The model under review builds one solid part; all positions refer to its coordinate system, in mm. Coordinates: 2 decimals unless noted, no trailing zeros. Loops run counter-clockwise (first coordinate to the right, second up) from the corner with the lowest first, then second, coordinate; pieces in that order, holes last. Notation, with made-up numbers: (-13.75, -37) -> (7.25, -37) arc R25 ccw to (7.25, -14) -> close; hole circle Ø3 at (-29, 32.25). An arc over 180 degrees is marked (long way). One line per question, with ' | ' between items. Start each with the question number.
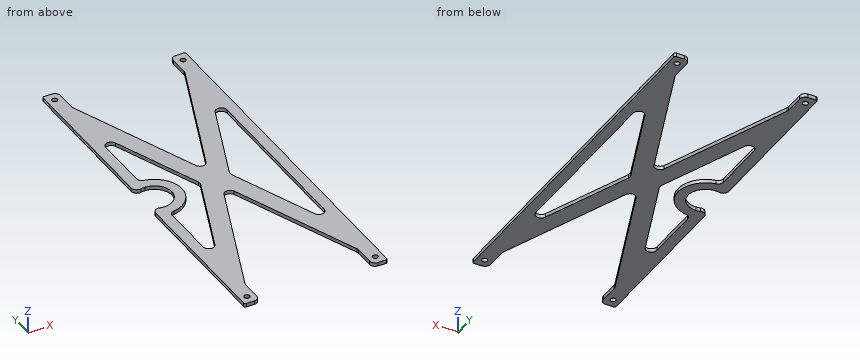
from build123d import *
from build123d.topology import SkipClean

# Parameters (mm, degrees)
EXTRUDE_1_DEPTH     = 2
SKETCH_4_R          = 1.5
CUT_EXTRUDE_3_DEPTH = 108.354552768
FILLET_4_R          = 1
CUT_EXTRUDE_5_DEPTH = 108.354552768
FILLET_7_R          = 3
EXTRUDE_2_DEPTH     = 2
CUT_EXTRUDE_6_DEPTH = 108.354552899
FILLET_8_R          = 3


with BuildPart() as part:
    # 草图1 → 凸台-拉伸1 (new body)
    with BuildSketch(Plane.XY):
        Polygon((39, 79.487179487), (33, 64.102564103), (33, -64.102564103), (39, -79.487179487), align=None)
        Polygon((33, -64.102564103), (8, 0), (0, -20.512820513), (31, -100), (39, -100), (39, -79.487179487), align=None)
        Polygon((-31, -100), (0, -20.512820513), (-8, 0), (-33, -64.102564103), (-39, -79.487179487), (-39, -100), align=None)
        Polygon((-33, -64.102564103), (-33, 64.102564103), (-39, 79.487179487), (-39, -79.487179487), align=None)
        Polygon((0, -20.512820513), (8, 0), (0, 20.512820513), (-8, 0), align=None)
        Polygon((8, 0), (33, 64.102564103), (39, 79.487179487), (39, 100), (31, 100), (0, 20.512820513), align=None)
        Polygon((-8, 0), (0, 20.512820513), (-31, 100), (-39, 100), (-39, 79.487179487), (-33, 64.102564103), align=None)
    extrude(amount=EXTRUDE_1_DEPTH)

    # 草图4 → 切除-拉伸3 (cut, through all)
    with BuildSketch(Plane.XY.offset(2)):
        with Locations((-35, 95)):
            Circle(SKETCH_4_R)
        with Locations(Location((-35, -95, 0), (0, 0, 180))):
            Circle(SKETCH_4_R)
        with Locations((35, -95)):
            Circle(SKETCH_4_R)
        with Locations(Location((35, 95, 0), (0, 0, 180))):
            Circle(SKETCH_4_R)
    extrude(amount=-CUT_EXTRUDE_3_DEPTH, mode=Mode.SUBTRACT)

    # 圆角4
    fillet_4_edges = [part.edges().sort_by_distance(p)[0] for p in [
        (39, -100, 1),
        (31, -100, 1),
        (-31, -100, 1),
        (-39, -100, 1),
        (-39, 100, 1),
        (-31, 100, 1),
        (31, 100, 1),
        (39, 100, 1),
    ]]
    fillet(fillet_4_edges, radius=FILLET_4_R)

    # 草图6 → 切除-拉伸5 (cut, through all)
    with BuildSketch(Plane.XY.offset(2)):
        Polygon((-30.751704658, -85.602329726), (-30.751704658, -99.363345276), (0, -20.512820513), (30.751704658, -99.363345276), (30.751704658, -85.602329726), (0, -6.751804962), align=None)
        Polygon((30.751704658, 85.602329726), (30.751704658, 99.363345276), (0, 20.512820513), (-30.751704658, 99.363345276), (-30.751704658, 85.602329726), (0, 6.751804962), align=None)
    extrude(amount=-CUT_EXTRUDE_5_DEPTH, mode=Mode.SUBTRACT)

    # 圆角7
    fillet_7_edges = [part.edges().sort_by_distance(p)[0] for p in [
        (30.751704658, 85.602329726, 1),
        (0, 6.751804962, 1),
        (-30.751704658, 85.602329726, 1),
        (-30.751704658, 99.363345276, 1),
        (-30.751704658, -99.363345276, 1),
        (0, -6.751804962, 1),
        (30.751704658, -85.602329726, 1),
        (30.751704658, -99.363345276, 1),
        (30.751704658, 99.363345276, 1),
        (33, 64.102564103, 1),
        (33, -64.102564103, 1),
        (8, 0, 1),
        (-8, 0, 1),
        (-33, -64.102564103, 1),
        (-33, 64.102564103, 1),
        (-30.751704658, -85.602329726, 1),
    ]]
    fillet(fillet_7_edges, radius=FILLET_7_R)

    # 草图7 → 凸台-拉伸2 (add, through all)
    with BuildSketch(Plane.XY.offset(2)):
        with BuildLine():
            ThreePointArc((-33, 9.5), (-26.282485579, 6.717514421), (-23.5, 0))
            ThreePointArc((-23.5, 0), (-26.282485579, -6.717514421), (-33, -9.5))
            Line((-33, -9.5), (-33, -15))
            ThreePointArc((-33, -15), (-22.393398282, -10.606601718), (-18, 0))
            ThreePointArc((-18, 0), (-22.393398282, 10.606601718), (-33, 15))
            Line((-33, 15), (-33, 9.5))
        make_face()
    extrude(amount=-EXTRUDE_2_DEPTH)

    # 草图7<4> → 切除-拉伸6 (cut, through all)
    with SkipClean():  # the faces are left unmerged after this step: merging them gives an invalid solid
        with BuildSketch(Plane.XY.offset(2)):
            with BuildLine():
                Line((-33, -9.5), (-33, 9.5))
                ThreePointArc((-33, 9.5), (-36.184189901, 8.950471198), (-39, 7.365459931))
                Line((-39, 7.365459931), (-39, -7.365459931))
                ThreePointArc((-39, -7.365459931), (-36.184189901, -8.950471198), (-33, -9.5))
            make_face()
        extrude(amount=-CUT_EXTRUDE_6_DEPTH, mode=Mode.SUBTRACT)

    # 圆角8
    fillet_8_edges = [part.edges().sort_by_distance(p)[0] for p in [
        (-33, -15, 1),
        (-33, 15, 1),
        (-39, -7.365459931, 1),
        (-39, 7.365459931, 1),
    ]]
    fillet(fillet_8_edges, radius=FILLET_8_R)


solid = part.part
1) Consider section A-A, the plane y = -53. Write out the cut boundary in (x, z).
2) Consider section C-C, the plane z = 0.8. Give the number of separate pieces and of enclosed holes in the cut face, plus the area to 3 significant figures.
3) Consider section B-B, the plane x = 23.5. Write out the cut boundary in (y, z), plus the area to 3 significant figures.
4) Wall thickness on L1, parallel to Y at x = 35, z = 1.5; L2, parallel to X at y = -95, z = 1.4; L3, parallel to X at y = 4, z = 0.2: over which ranges is each line inside the solid? List them lowest first.
5) Consider section D-D, the plane x = -6.5. Write out the cut boundary in (y, z).
Filled sheet:
1) outline: (-39, 0) -> (-18.04, 0) -> (-18.04, 2) -> (-39, 2) -> close; (18.04, 0) -> (39, 0) -> (39, 2) -> (18.04, 2) -> close
2) separate pieces: 1 | enclosed holes: 6 | area: 6,000 mm^2
3) outline: (-67.01, 0) -> (-39.74, 0) -> (-39.74, 2) -> (-67.01, 2) -> close; (39.74, 0) -> (67.01, 0) -> (67.01, 2) -> (39.74, 2) -> close | area: 109 mm^2
4) L1: -100 to -96.5, -93.5 to 93.5, 96.5 to 100 | L2: -39 to -36.5, -33.5 to -30.75, 30.75 to 33.5, 36.5 to 39 | L3: -24.38 to -18.54, -9.56 to 9.56, 33 to 39
5) outline: (-23.42, 0) -> (23.42, 0) -> (23.42, 2) -> (-23.42, 2) -> close
